Geometry: final body of the model. Coordinates: model frame, mm. Face numbers are marked on the shaded views. A direction names the side the tool comes from. Give positions to 0.01 mm unless a question says otherwise; leave off trailing zeros. Loops run counter-clockwise (first coordinate to the right, second up) from the corner with the lowest first, then second, coordinate; pieces in that order, holes last. Notation, with made-up numbers: (38, 67) -> (50, 67) arc R29 ccw to (50, 90) -> close; hole circle Ø11 at (54.25, 7). An arc over 180 degrees is marked (long way). Answer in a Markdown table with one row per item. Add a question column.
1) Access query for the marked faces 1, 2, 3, 4 and 5. Directions: +Z, -Z, +X, -X, +Y, -Y. A direction counts if a zero-diameter tool reaches every point of the face in a straight line with its end or side. Return the directions, or none.
2) Line query: line 1 (Y direction, x = 131.5, z = 21.5); line 2 (Z direction, x = 95.5, y = 69); line 3 (Z direction, x = 53.5, y = 64). Output: solid intervals per line, ascending. Write a range as from..to.
3) Draft query along X for the marked faces 6, 7 and 8. Return one class per face: +X half, -X half, draft (parallel to the pull), parting line (faces both ways), or undercut.
4) Section query B-B (z = 37). Return the cut outline in (x, y).
5) Section query A-A (y = 60). Return the cut outline in (x, z), plus the area to 3 significant figures.
6) First-contact query: P1, Ø8, axis at x = 94, z = 37, coming from the -Y side; P2, Ø9, axis at y = 59, z = 18.5, coming from the -X side; P3, Ø16, axis at y = 108.5, z = 19, coming from the -X side; P4, Ø6, axis at y = 79, z = 12, coming from the +X side. Flat tips, straight axial feed; report the tip coordinate or a pass-through.
7) Section query C-C (z = 14). Return the cut outline in (x, y), plus the area to 3 significant figures.
8) Section query D-D (x = 112). Return the cut outline in (y, z), plus the area to 3 significant figures.
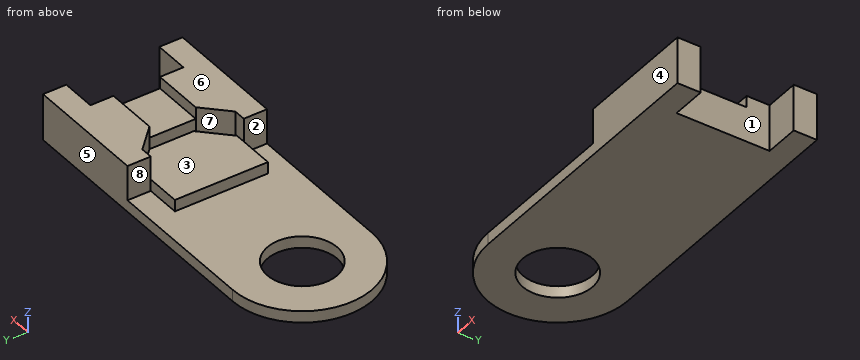
```python
from build123d import *

# Parameters (mm, degrees)
SKETCH2_R           = 30
BOSS_EXTRUDE2_DEPTH = 10
SKETCH4_W           = 39.74410588
SKETCH4_H           = 80
CUT_EXTRUDE1_DEPTH  = 30
SKETCH5_W           = 105
SKETCH5_H           = 120
BOSS_EXTRUDE3_DEPTH = 40
SKETCH6_W           = 78.106224714
SKETCH6_H           = 80
CUT_EXTRUDE2_DEPTH  = 30
SKETCH7_W           = 45
SKETCH7_H           = 40
CUT_EXTRUDE3_DEPTH  = 10
CUT_EXTRUDE4_DEPTH  = 30
BOSS_EXTRUDE4_DEPTH = 10


with BuildPart() as part:
    # Sketch2 → Boss-Extrude2 (new body)
    with BuildSketch(Plane.XY):
        with BuildLine():
            Line((46.207044142, 120), (-84.343419201, 120))
            ThreePointArc((-84.343419201, 120), (-144.343419201, 60), (-84.343419201, 0))
            Line((-84.343419201, 0), (0, 0))
            Line((0, 0), (151.207044142, 0))
            Line((151.207044142, 0), (151.207044142, 120))
            Line((151.207044142, 120), (46.207044142, 120))
        make_face()
        with Locations((-84.343419201, 60)):
            Circle(SKETCH2_R, mode=Mode.SUBTRACT)
    extrude(amount=BOSS_EXTRUDE2_DEPTH)

    # Sketch4 → Cut-Extrude1 (cut)
    with BuildSketch(Plane(origin=(151.207044142, 0, 0), x_dir=(0, 0, -1), z_dir=(1, 0, 0))):
        with Locations((-1.423296347, 60)):
            Rectangle(SKETCH4_W, SKETCH4_H)
    extrude(amount=-CUT_EXTRUDE1_DEPTH, mode=Mode.SUBTRACT)

    # Sketch5 → Boss-Extrude3 (add)
    with BuildSketch(Plane.XY):
        with Locations((98.707044142, 60)):
            Rectangle(SKETCH5_W, SKETCH5_H)
    extrude(amount=BOSS_EXTRUDE3_DEPTH)

    # Sketch6 → Cut-Extrude2 (cut)
    with BuildSketch(Plane(origin=(151.207044142, 0, 0), x_dir=(0, 0, -1), z_dir=(1, 0, 0))):
        with Locations((-16.932746975, 60)):
            Rectangle(SKETCH6_W, SKETCH6_H)
    extrude(amount=-CUT_EXTRUDE2_DEPTH, mode=Mode.SUBTRACT)

    # Sketch7 → Cut-Extrude3 (cut)
    with BuildSketch(Plane.XY.offset(40)):
        with Locations((99.042729198, 60.209092216)):
            Rectangle(SKETCH7_W, SKETCH7_H)
    extrude(amount=-CUT_EXTRUDE3_DEPTH, mode=Mode.SUBTRACT)

    # Sketch8 → Cut-Extrude4 (cut)
    with BuildSketch(Plane.XY.offset(40)):
        Polygon((19.599086243, 100), (56.633635385, 100), (76.633635385, 80), (76.633635385, 40), (56.633635385, 20), (19.599086243, 20), align=None)
    extrude(amount=-CUT_EXTRUDE4_DEPTH, mode=Mode.SUBTRACT)

    # Sketch9 → Boss-Extrude4 (add)
    with BuildSketch(Plane.XY.offset(10)):
        Polygon((46.207044142, 100), (16.207044142, 100), (16.207044142, 20), (46.207044142, 20), (54.69343027, 20), (76.633635385, 41.940205115), (76.633635385, 80), (56.633635385, 100), align=None)
    extrude(amount=BOSS_EXTRUDE4_DEPTH)


solid = part.part
```
Evaluation:
| question | item | result |
|---|---|---|
| 1 | face 1 | +Z, -Z, +X |
| 1 | face 2 | +Z, -X, -Y |
| 1 | face 3 | +Z, -X |
| 1 | face 4 | +Z, -Z, +X, -X, -Y |
| 1 | face 5 | +Z, -Z, +X, -X, +Y |
| 2 | line 1 | 0..20, 100..120 |
| 2 | line 2 | 0..30 |
| 2 | line 3 | 0..20 |
| 3 | face 6 | draft |
| 3 | face 7 | undercut |
| 3 | face 8 | -X half |
| 4 | outline | (46.21, 0) -> (151.21, 0) -> (151.21, 20) -> (121.21, 20) -> (121.21, 40.21) -> (76.63, 40.21) -> (76.63, 40) -> (56.63, 20) -> (46.21, 20) -> close; (46.21, 100) -> (56.63, 100) -> (76.54, 80.09) -> (76.54, 80.21) -> (121.21, 80.21) -> (121.21, 100) -> (151.21, 100) -> (151.21, 120) -> (46.21, 120) -> close |
| 5 | outline | (-144.34, 0) -> (-114.34, 0) -> (-114.34, 10) -> (-144.34, 10) -> close; (-54.34, 0) -> (121.21, 0) -> (121.21, 30) -> (76.63, 30) -> (76.63, 20) -> (16.21, 20) -> (16.21, 10) -> (-54.34, 10) -> close |
| 5 | area | 3,550 mm² |
| 6 | P1 | y = 0 |
| 6 | P2 | x = 16.21 |
| 6 | P3 | x = 46.21 |
| 6 | P4 | x = 121.21 |
| 7 | outline | (16.21, 20) -> (46.21, 20) -> (46.21, 0) -> (151.21, 0) -> (151.21, 20) -> (121.21, 20) -> (121.21, 100) -> (151.21, 100) -> (151.21, 120) -> (46.21, 120) -> (46.21, 100) -> (16.21, 100) -> close; hole (54.69, 20) -> (56.63, 20) -> (76.63, 40) -> (76.63, 41.94) -> close |
| 7 | area | 12,600 mm² |
| 8 | outline | (0, 0) -> (120, 0) -> (120, 40) -> (80.21, 40) -> (80.21, 30) -> (40.21, 30) -> (40.21, 40) -> (0, 40) -> close |
| 8 | area | 4,400 mm² |
